from build123d import *

# Parameters (mm, degrees)
F1_DEPTH = 4.7625
F2_R     = 14.351
F3_DEPTH = 21.336
F4_DEPTH = 10.16
F2_W     = 70.104
F2_H     = 44.958
F5_DEPTH = 15.24
F2_W_2   = 53.570382297
F2_H_2   = 30.4797645658
F6_DEPTH = 17.78
F7_SCALE = 0.96


with BuildPart() as f1:
    # F0 (on Top) → F1 (new body)
    with BuildSketch(Plane.XY):
        with BuildLine():
            ThreePointArc((-55.5763468146, 79.3343931437), (-90.9271049645, 108.8918614568), (-122.7753036062, 142.1936974142))
            ThreePointArc((-122.7753036062, 142.1936974142), (-147.9363073453, 147.9363073453), (-142.1936974142, 122.7753036062))
            ThreePointArc((-142.1936974142, 122.7753036062), (-108.8918614568, 90.9271049645), (-79.3343931437, 55.5763468146))
            ThreePointArc((-79.3343931437, 55.5763468146), (-72.3967482518, 0), (-79.3343931437, -55.5763468146))
            ThreePointArc((-79.3343931437, -55.5763468146), (-108.8918614568, -90.9271049645), (-142.1936974142, -122.7753036062))
            ThreePointArc((-142.1936974142, -122.7753036062), (-147.9363073453, -147.9363073453), (-122.7753036062, -142.1936974142))
            ThreePointArc((-122.7753036062, -142.1936974142), (-90.9271049645, -108.8918614568), (-55.5763468146, -79.3343931437))
            ThreePointArc((-55.5763468146, -79.3343931437), (0, -72.3967482518), (55.5763468146, -79.3343931437))
            ThreePointArc((55.5763468146, -79.3343931437), (90.9271049645, -108.8918614568), (122.7753036062, -142.1936974142))
            ThreePointArc((122.7753036062, -142.1936974142), (147.9363073453, -147.9363073453), (142.1936974142, -122.7753036062))
            ThreePointArc((142.1936974142, -122.7753036062), (108.8918614568, -90.9271049645), (79.3343931437, -55.5763468146))
            ThreePointArc((79.3343931437, -55.5763468146), (72.3967482518, 0), (79.3343931437, 55.5763468146))
            ThreePointArc((79.3343931437, 55.5763468146), (108.8918614568, 90.9271049645), (142.1936974142, 122.7753036062))
            ThreePointArc((142.1936974142, 122.7753036062), (147.9363073453, 147.9363073453), (122.7753036062, 142.1936974142))
            ThreePointArc((122.7753036062, 142.1936974142), (90.9271049645, 108.8918614568), (55.5763468146, 79.3343931437))
            ThreePointArc((55.5763468146, 79.3343931437), (0, 72.3967482518), (-55.5763468146, 79.3343931437))
        make_face()
        Polygon((-115.2469329536, -119.5561625063), (-119.5561625063, -115.2469329536), (-87.3443447053, -83.0351151526), (-83.0351151526, -87.3443447053), align=None, mode=Mode.SUBTRACT)
        Polygon((115.2469329536, -119.5561625063), (83.0351151526, -87.3443447053), (87.3443447053, -83.0351151526), (119.5561625063, -115.2469329536), align=None, mode=Mode.SUBTRACT)
        Polygon((-119.5561625063, 115.2469329536), (-117.40154773, 117.40154773), (-115.2469329536, 119.5561625063), (-83.0351151526, 87.3443447053), (-85.189729929, 85.189729929), (-87.3443447053, 83.0351151526), align=None, mode=Mode.SUBTRACT)
        Polygon((87.3443447053, 83.0351151526), (83.0351151526, 87.3443447053), (115.2469329536, 119.5561625063), (119.5561625063, 115.2469329536), align=None, mode=Mode.SUBTRACT)
    extrude(amount=F1_DEPTH)

    # F2 (on face) → F3 (join)
    with BuildSketch(Plane.XY.offset(4.7625)):
        with Locations((-137.16, 137.16)):
            Circle(F2_R)
        with Locations((137.16, 137.16)):
            Circle(F2_R)
        with Locations((137.16, -137.16)):
            Circle(F2_R)
        with Locations((-137.16, -137.16)):
            Circle(F2_R)
    extrude(amount=F3_DEPTH)

    # F2 (on face) → F4 (join)
    with BuildSketch(Plane.XY.offset(4.7625)):
        Polygon((-108.3536930382, 118.1755252182), (-111.1099943519, 115.4192239046), (-94.6341976523, 98.9434272051), (-91.8778963387, 101.6997285187), align=None)
        Polygon((-111.1099943519, 115.4192239046), (-113.2646091282, 113.2646091282), (-115.4192239046, 111.1099943519), (-98.9434272051, 94.6341976523), (-96.7888124287, 96.7888124287), (-94.6341976523, 98.9434272051), align=None)
        Polygon((-98.9434272051, 94.6341976523), (-115.4192239046, 111.1099943519), (-118.1755252182, 108.3536930382), (-101.6997285187, 91.8778963387), align=None)
        Polygon((118.1755252182, 108.3536930382), (115.4192239046, 111.1099943519), (98.9434272051, 94.6341976523), (101.6997285187, 91.8778963387), align=None)
        Polygon((115.4192239046, 111.1099943519), (113.2646091282, 113.2646091282), (111.1099943519, 115.4192239046), (94.6341976523, 98.9434272051), (96.7888124287, 96.7888124287), (98.9434272051, 94.6341976523), align=None)
        Polygon((94.6341976523, 98.9434272051), (111.1099943519, 115.4192239046), (108.3536930382, 118.1755252182), (91.8778963387, 101.6997285187), align=None)
        Polygon((91.8778963387, -101.6997285187), (108.3536930382, -118.1755252182), (111.1099943519, -115.4192239046), (94.6341976523, -98.9434272051), align=None)
        Polygon((94.6341976523, -98.9434272051), (111.1099943519, -115.4192239046), (113.2646091282, -113.2646091282), (115.4192239046, -111.1099943519), (98.9434272051, -94.6341976523), (96.7888124287, -96.7888124287), align=None)
        Polygon((98.9434272051, -94.6341976523), (115.4192239046, -111.1099943519), (118.1755252182, -108.3536930382), (101.6997285187, -91.8778963387), align=None)
        Polygon((-98.9434272051, -94.6341976523), (-101.6997285187, -91.8778963387), (-118.1755252182, -108.3536930382), (-115.4192239046, -111.1099943519), align=None)
        Polygon((-96.7888124287, -96.7888124287), (-98.9434272051, -94.6341976523), (-115.4192239046, -111.1099943519), (-113.2646091282, -113.2646091282), (-111.1099943519, -115.4192239046), (-94.6341976523, -98.9434272051), align=None)
        Polygon((-91.8778963387, -101.6997285187), (-94.6341976523, -98.9434272051), (-111.1099943519, -115.4192239046), (-108.3536930382, -118.1755252182), align=None)
    extrude(amount=F4_DEPTH)

    # F2 (on face) → F5 (join)
    with BuildSketch(Plane.XY.offset(4.7625)):
        with Locations((0, 38.2346063852)):
            Rectangle(F2_W, F2_H)
    extrude(amount=F5_DEPTH)

    # F2 (on face) → F6 (join)
    with BuildSketch(Plane.XY.offset(4.7625)):
        with Locations((0, -28.266698122)):
            Rectangle(F2_W_2, F2_H_2)
    extrude(amount=F6_DEPTH)


with BuildPart() as f1_1:
    # F7: moved
    add(f1.part.scale(F7_SCALE))


solid = f1_1.part
Can you work these out from the model? Positions are in its coordinate system, mm. A direction names the side the tool comes from. Give positions to 0.01 mm unless a question says otherwise; leave off trailing zeros. Order: outer loops, then holes, each group sorted by start corner. A loop starts at its lowest first (then second) coordinate and runs counter-clockwise, first axis right, second up. Notation, with made-up numbers: M 66.25,40 L 108.25,40 A30 cw 108.25,68 Z; hole C 55.25,47.5 d7. An arc over 180 degrees is marked long. Use one line per item in the form item = value. Start each with the question number.
Item 1: If we section it at C-C (y = -35): Write out the boundary of the cut face in (x, z).
Item 2: We'd pull the mould along Y, two halves only. Please class faces 1 (the cylindrical face through (-141.72, 142.31, 2.25)), 2 (the flat face through (-96.22, -105.65, 9.38)), 3 (the flat face through (25.714, -27, 13)): +Y half, -Y half, draft (parallel to the pull), parting line (faces both ways), or undercut.
Item 3: Will these pins go through, and if not, where does the flat tip stop? pin 1 Ø12.5 at (x, y) = (-102.5, 96.5) entering from +Z; pin 2 Ø13.5 at (x, z) = (8.5, 14.5) entering from -Y; pin 3 Ø11.5 at (y, z) = (31.5, 9.5) entering from -X.
Item 4: For faces 4 (the flat face through (-94.959, -99.096, 2.254)), 5 (the cylindrical face through (104.113, 86.837, 2.254)), 6 (the flat face through (-33.65, 36, 12)), 7 (the flat face through (92.983, -92.851, 9.381)), 8 (the flat face through (0, 58.285, 12)), which set-ups out of +Z, -Z, +X, -X, +Y, -Y let a thin tool reach every point of the face, with its end or its side?
Item 5: If we section it at D-D (x = 63.5): Write out the boundary of the cut face in (y, z).
Item 6: If we section it at A-A (y = 46): Write out the boundary of the cut face in (x, z), then the cut area to 3 significant figures.
Item 7: If I drill on line 1 along X through (y, z) = (-96, 3); line 2 along X through (y, z) = (-132.5, 11.5); line 3 along Y through (x, z) = (-131, 6.75), over which ranges is the centre line in solid material (lowest first)?
Item 8: If we section it at B-B (x = 3): Write out the boundary of the cut face in (y, z), then the cut area to 3 significant figures.
Outcome:
q1.outline = M -72.34,0 L 72.34,0 L 72.34,4.57 L 25.71,4.57 L 25.71,21.64 L -25.71,21.64 L -25.71,4.57 L -72.34,4.57 Z
q2.face_1 = undercut
q2.face_2 = -Y half
q2.face_3 = draft
q3.pin_1 = 14.33
q3.pin_2 = -41.77
q3.pin_3 = -72.25
q4.face_4 = -Z
q4.face_5 = +Z, -Z, +X
q4.face_6 = +Z, -X, +Y, -Y
q4.face_7 = +Z
q4.face_8 = +Z, +X, -X, +Y
q5.outline = M -83.98,0 L 83.98,0 L 83.98,4.57 L -83.98,4.57 Z
q6.outline = M -74.43,0 L 74.43,0 L 74.43,4.57 L 33.65,4.57 L 33.65,19.2 L -33.65,19.2 L -33.65,4.57 L -74.43,4.57 Z
q6.area = 1,670 mm2
q7.line_1 = -112.94 to -100.14, -91.86 to -77.87, 77.87 to 91.86, 100.14 to 112.94
q7.line_2 = -145.43 to -117.92, 117.92 to 145.43
q7.line_3 = -145.43 to -117.91, 117.91 to 145.43
q8.outline = M -69.52,0 L 69.52,0 L 69.52,4.57 L 58.29,4.57 L 58.29,19.2 L 15.13,19.2 L 15.13,4.57 L -12.51,4.57 L -12.51,21.64 L -41.77,21.64 L -41.77,4.57 L -69.52,4.57 Z
q8.area = 1,770 mm2
